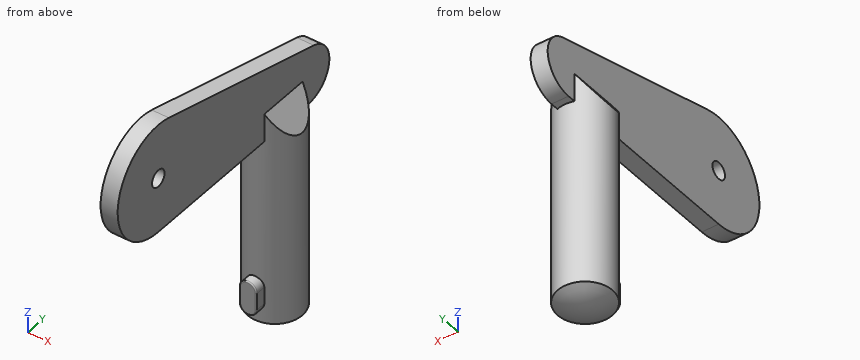
from build123d import *

# Parameters (mm, degrees)
F0_R          = 4.825
F1_DEPTH      = 33
F3_DEPTH      = 6.5
F4_R          = 0.2
F8_DEPTH      = 1.5
F8_DEPTH_BACK = 1.5
F9_T4_DEPTH   = 34.9974315038
F9_S5_R       = 4.825
F9_T6_DEPTH   = 19
F9_T10_DEPTH  = 34.9974315038
F9_S11_R      = 4.825
F9_T12_DEPTH  = 19
F11_R         = 1.5
F12_DEPTH     = 6.3260001


# Not quite as in the source:
# - a fillet or chamfer that OpenCascade refuses, or shapes differently, is made with other operations: its cross-section is extruded or revolved along the edge and cut away or added
# - a feature of the source that left no trace in its solid (it failed there, or was rolled back) is left out


with BuildPart() as f1:
    # F0 (on Top) → F1 (new body)
    with BuildSketch(Plane.XY):
        Circle(F0_R)
    extrude(amount=F1_DEPTH)

    # F2 (on Front) → F3 (join)
    with BuildSketch(Plane.XZ):
        with BuildLine():
            ThreePointArc((-1.5, 3.5), (0, 2), (1.5, 3.5))
            Line((1.5, 3.5), (1.5, 6.5))
            ThreePointArc((1.5, 6.5), (0, 8), (-1.5, 6.5))
            Line((-1.5, 6.5), (-1.5, 3.5))
        make_face()
    extrude(amount=F3_DEPTH)

    # F4
    f4_edges = [f1.edges().sort_by_distance(p)[0] for p in [
        (0, -6.5, 2),
        (1.5, -6.5, 5),
        (0, -6.5, 8),
        (-1.5, -6.5, 5),
    ]]
    fillet(f4_edges, radius=F4_R)

    # F5 (on Front) → F6 (revolve)
    with BuildSketch(Plane.XZ):
        with BuildLine():
            Line((0, 0), (-4.825, 0))
            ThreePointArc((-4.825, 0), (-2.5263919431, -1.1163524169), (0, -1.5))
            Line((0, -1.5), (0, 0))
        make_face()
    revolve(axis=Axis((0, 0, -1.4078605181), (0, 0, -1)))

    # F7 (on Right) → F8 (join, two sides)
    with BuildSketch(Plane.YZ) as f8_sk:
        with BuildLine():
            ThreePointArc((6, 33), (10.9572243069, 37.3473690389), (7.2940952255, 42.8296291314))
            Line((7.2940952255, 42.8296291314), (-27.4792345209, 52.1471147551))
            ThreePointArc((-27.4792345209, 52.1471147551), (-39.6561672268, 44.0107484457), (-30, 33))
            Line((-30, 33), (-6, 33))
            Line((-6, 33), (6, 33))
        make_face()
    extrude(amount=F8_DEPTH)
    extrude(f8_sk.sketch, amount=-F8_DEPTH_BACK)

    # F9: chamfer of 3.5 x 5 on 2 edges, made by hand


with BuildPart() as f9_tool2:
    # F9_s3 → F9_t4 (new body)
    with BuildSketch(Plane.XZ.offset(-17.4987157519)):
        Polygon((5, 33), (1.5, 38), (1.5, 33), align=None)
    extrude(amount=F9_T4_DEPTH)

    # F9_s5 → F9_t6 (intersect, symmetric)
    with BuildSketch(Plane.XY.offset(35.5)):
        Circle(F9_S5_R)
    extrude(amount=F9_T6_DEPTH, both=True, mode=Mode.INTERSECT)


with BuildPart() as f1_1:
    add(f1.part)

    # F9_t1: union F9_tool2
    add(f9_tool2.part)


with BuildPart() as f9_tool8:
    # F9_s9 → F9_t10 (new body)
    with BuildSketch(Plane.XZ.offset(17.4987157519)):
        Polygon((-5, 33), (-1.5, 38), (-1.5, 33), align=None)
    extrude(amount=-F9_T10_DEPTH)

    # F9_s11 → F9_t12 (intersect, symmetric)
    with BuildSketch(Plane.XY.offset(35.5)):
        Circle(F9_S11_R)
    extrude(amount=F9_T12_DEPTH, both=True, mode=Mode.INTERSECT)


with BuildPart() as f1_2:
    add(f1_1.part)

    # F9_t7: union F9_tool8
    add(f9_tool8.part)

    # F11 (on face) → F12 (cut, through all)
    with BuildSketch(Plane.YZ.offset(1.5)):
        with Locations((-30, 42.7394899131)):
            Circle(F11_R)
    extrude(amount=-F12_DEPTH, mode=Mode.SUBTRACT)


solid = f1_2.part
Here's how the part is built. I have some questions about the finished solid (model axes, mm). Coordinates: 2 decimals unless noted, no trailing zeros. Order: outer loops, then holes, each group sorted by start corner. A loop starts at its lowest first (then second) coordinate and runs counter-clockwise, first axis right, second up. Notation, with made-up numbers: (-28, -27.75) -> (17, -27.75) arc R13 ccw to (17, -8.75) -> close; hole circle Ø11 at (-31.75, 11). An arc over 180 degrees is marked (long way). Answer in a Markdown table with one row per item.
(1) I want a section at A-A on x = 0. List the corners of the cut face in (y, z) for me (3 decimals).
Answer key:
| item | result |
|---|---|
| outline | (-30, 33) -> (-4.825, 33) -> (-4.825, 8) -> (-6.3, 8) arc R0.2 ccw to (-6.5, 7.8) -> (-6.5, 2.2) arc R0.2 ccw to (-6.3, 2) -> (-4.825, 2) -> (-4.825, 0) arc R8.51 ccw to (4.825, 0) -> (4.825, 33) -> (6, 33) arc R5 ccw to (7.294, 42.83) -> (-27.479, 52.147) arc R9.739 ccw (long way) to start; hole circle Ø3 at (-30, 42.739) |
(2) Please list where these lines run through material, in increasing order: probe 1 along Z at (x, y) = (0.1, -30); probe 2 along X at (y, z) = (-19.5, 40); probe 3 along Y at (x, z) = (-1.5, 16.5).
Answer key:
| item | result |
|---|---|
| probe 1 | 33 to 41.24, 44.24 to 52.48 |
| probe 2 | -1.5 to 1.5 |
| probe 3 | -4.59 to 4.59 |
(3) I want a section at D-D on x = -3. List the corners of the cut face in (y, z) for me.
Answer key:
| item | result |
|---|---|
| outline | (-3.78, 0) arc R7.96 ccw to (3.78, 0) -> (3.78, 35.86) -> (-3.78, 35.86) -> close |
(4) I want a section at B-B on z = 25. List the corners of the cut face in (x, y) for me (3 decimals), then the cut area to 3 significant figures.
Answer key:
| item | result |
|---|---|
| outline | circle Ø9.65 at (0, 0) |
| area | 73.1 mm^2 |
(5) Will these pins go through, and if not, where does the flat tip stop? pin 1 Ø0.9 at (y, z) = (-5.5, 5.5) entering from +X; pin 2 Ø9.5 at (y, z) = (-9, 47) entering from -X; pin 3 Ø2 at (x, z) = (-2, 11.5) entering from +Y.
Answer key:
| item | result |
|---|---|
| pin 1 | x = 1.5 |
| pin 2 | x = -1.5 |
| pin 3 | y = 4.72 |
(6) I want a section at C-C on y = -20. List the corners of the cut face in (x, z) for me.
Answer key:
| item | result |
|---|---|
| outline | (-1.5, 33) -> (1.5, 33) -> (1.5, 50.14) -> (-1.5, 50.14) -> close |
